Could you check a few things on this drawing? It's one solid part, dimensions in mm from its lowest x, y, z. Round coordinates to 2 decimals unless told otherwise and drop trailing zeros. Loops run counter-clockwise (first coordinate to the right, second up) from the corner with the lowest first, then second, coordinate; pieces in that order, holes last. Notation, with made-up numbers: (31.25, -9.75) -> (55.25, -9.75) arc R14 ccw to (55.25, 4.25) -> close; hole circle Ø1 at (49, 59). An arc over 180 degrees is marked (long way). Use one line per item in the form item = value. Start each with the question number.
Item 1: If we section it at A-A (z = 50.5): Write out the boundary of the cut face in (x, y).
Item 2: I'm going to push a flat-ended pin straight in: pin 1 Ø21 at (x, z) = (24, 21.51) entering from +Y. Where does the tip first touch, or does it pass through?
Item 3: If I drill on L1, parallel to Z at x = 24, y = 3.7 (1 decimal); L2, parallel to Z at x = 22.5, y = 1; L3, parallel to Y at x = 22.5, z = 71, over which ranges is the centre line in solid material (lowest first)? Write a range as [from, to].
Item 4: If we section it at B-B (x = 24): Write out the boundary of the cut face in (y, z) (1 decimal), then the cut area to 3 significant figures.
Item 5: If we section it at D-D (z = 26): Write out the boundary of the cut face in (x, y), then the cut area to 3 significant figures.
Item 6: If we section it at C-C (y = 4): Write out the boundary of the cut face in (x, z) (1 decimal), then the cut area to 3 significant figures.
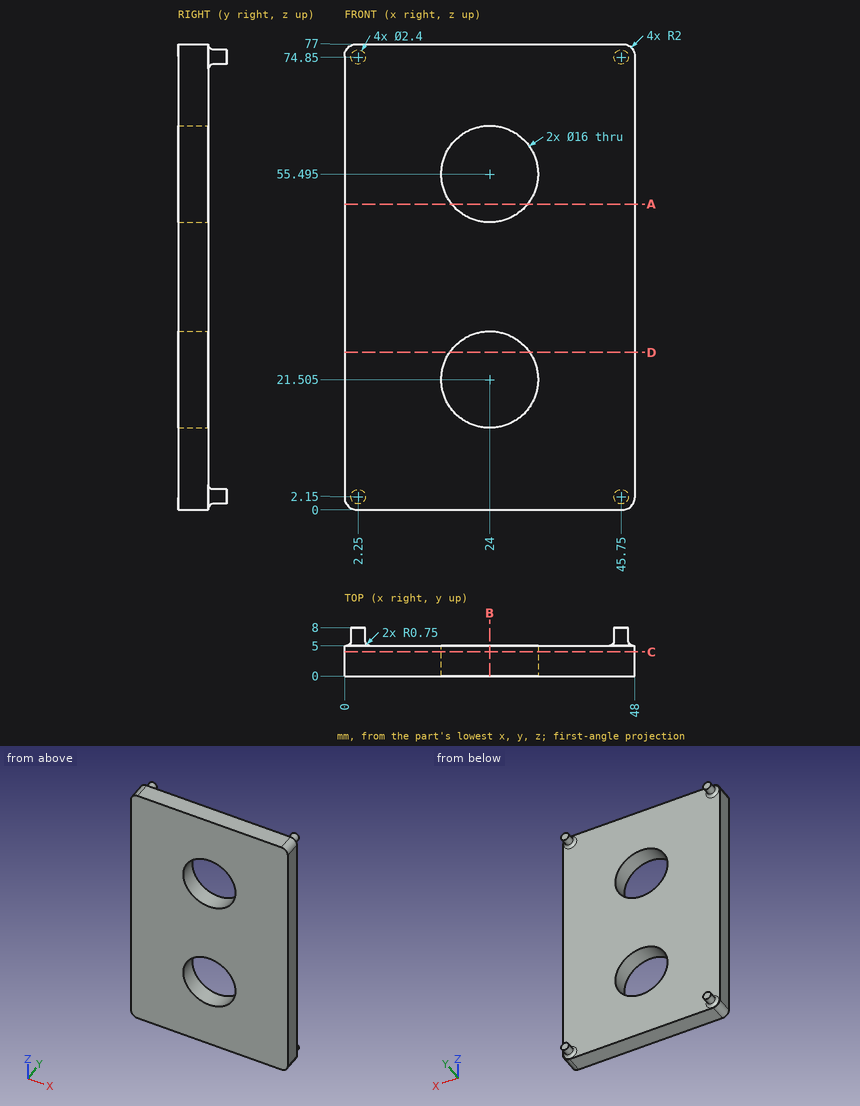
Values found:
q1.outline = (0, 0) -> (17.75, 0) -> (17.75, 5) -> (0, 5) -> close; (30.25, 0) -> (48, 0) -> (48, 5) -> (30.25, 5) -> close
q2.pin_1 = 5
q3.L1 = [0, 13.5], [29.5, 47.5], [63.5, 77]
q3.L2 = [0, 13.65], [29.36, 47.64], [63.35, 77]
q3.L3 = [0, 5]
q4.outline = (0, 0) -> (5, 0) -> (5, 13.5) -> (0, 13.5) -> close; (0, 29.5) -> (5, 29.5) -> (5, 47.5) -> (0, 47.5) -> close; (0, 63.5) -> (5, 63.5) -> (5, 77) -> (0, 77) -> close
q4.area = 225 mm2
q5.outline = (0, 0) -> (17.38, 0) -> (17.38, 5) -> (0, 5) -> close; (30.62, 0) -> (48, 0) -> (48, 5) -> (30.62, 5) -> close
q5.area = 174 mm2
q6.outline = (0, 2) arc R2 ccw to (2, 0) -> (46, 0) arc R2 ccw to (48, 2) -> (48, 75) arc R2 ccw to (46, 77) -> (2, 77) arc R2 ccw to (0, 75) -> close; hole circle Ø16 at (24, 21.5); hole circle Ø16 at (24, 55.5)
q6.area = 3,290 mm2
